```python
from build123d import *

# Parameters (mm, degrees)
SKETCH2_W            = 483.00005
SKETCH2_H            = 88.0999
BOSS_EXTRUDE2_DEPTH  = 3.0988
SKETCH3_W            = 163.4007
SKETCH3_H            = 30.8991
CUT_EXTRUDE1_DEPTH   = 3.0988
SKETCH5_R            = 2.5
CUT_EXTRUDE2_DEPTH   = 9.1948
LPATTERN1_COUNT      = 6
LPATTERN1_PITCH      = 20.32
LPATTERN1_COUNT_DIR2 = 4
LPATTERN1_PITCH_DIR2 = 10.16
SKETCH6_R            = 6.5024
CUT_EXTRUDE3_DEPTH   = 9.1948
LPATTERN2_COUNT      = 8
LPATTERN2_PITCH      = 20.32
SKETCH7_R            = 6.5024
CUT_EXTRUDE4_DEPTH   = 491.978862316
SKETCH8_R            = 5.92074
CUT_EXTRUDE5_DEPTH   = 491.978862316
SKETCH9_R            = 1.999996
CUT_EXTRUDE6_DEPTH   = 491.978862316
LPATTERN3_COUNT      = 6
LPATTERN3_PITCH      = 20.32
SKETCH10_R           = 2.5
CUT_EXTRUDE7_DEPTH   = 491.978862316
LPATTERN4_COUNT      = 2
LPATTERN4_PITCH      = 25.4
LPATTERN4_COUNT_DIR2 = 4
LPATTERN4_PITCH_DIR2 = 15.24
SKETCH11_R           = 1.999996
CUT_EXTRUDE8_DEPTH   = 491.978862316
LPATTERN5_COUNT      = 4
LPATTERN5_PITCH      = 10.16
SKETCH12_R           = 1.75
CUT_EXTRUDE9_DEPTH   = 491.978862316
LPATTERN6_COUNT      = 2
LPATTERN6_PITCH      = 12.7
LPATTERN6_COUNT_DIR2 = 2
LPATTERN6_PITCH_DIR2 = 25.4
SKETCH13_R           = 1.999996
CUT_EXTRUDE10_DEPTH  = 491.978862316
SKETCH15_R           = 5.92074
CUT_EXTRUDE11_DEPTH  = 491.978862316
LPATTERN7_COUNT      = 4
LPATTERN7_PITCH      = 38.1
SKETCH16_R           = 1.4732
CUT_EXTRUDE12_DEPTH  = 491.978862316
SKETCH17_R           = 1.4732
CUT_EXTRUDE13_DEPTH  = 491.978862316
SKETCH18_R           = 1.4732
CUT_EXTRUDE14_DEPTH  = 491.978862316


with BuildPart() as part:
    # Sketch2 → Boss-Extrude2 (new body)
    with BuildSketch(Plane.XY):
        with Locations((241.500025, 44.04995)):
            Rectangle(SKETCH2_W, SKETCH2_H)
    extrude(amount=-BOSS_EXTRUDE2_DEPTH)

    # Sketch3 → Cut-Extrude1 (cut)
    with BuildSketch(Plane.XY):
        with Locations((175.887888, 65.19037)):
            Rectangle(SKETCH3_W, SKETCH3_H)
    extrude(amount=-CUT_EXTRUDE1_DEPTH, mode=Mode.SUBTRACT)

    # Sketch5 → Cut-Extrude2 (cut)
    with BuildSketch(Plane.XY):
        with Locations((310.52008, 75.3999)):
            Circle(SKETCH5_R)
    cut_extrude2 = extrude(amount=-CUT_EXTRUDE2_DEPTH, mode=Mode.SUBTRACT)

    # LPattern1: Cut-Extrude2 6 × 4
    with Locations(*[(i * LPATTERN1_PITCH, -j * LPATTERN1_PITCH_DIR2, 0) for i in range(LPATTERN1_COUNT) for j in range(LPATTERN1_COUNT_DIR2) if (i, j) != (0, 0)]):
        add(cut_extrude2, mode=Mode.SUBTRACT)

    # Sketch6 → Cut-Extrude3 (cut)
    with BuildSketch(Plane.XY):
        with Locations((104.78008, 30.48)):
            Circle(SKETCH6_R)
    cut_extrude3 = extrude(amount=-CUT_EXTRUDE3_DEPTH, mode=Mode.SUBTRACT)

    # LPattern2: Cut-Extrude3 ×8
    with Locations(*[(i * LPATTERN2_PITCH, 0, 0) for i in range(1, LPATTERN2_COUNT)]):
        add(cut_extrude3, mode=Mode.SUBTRACT)

    # Sketch7 → Cut-Extrude4 (cut, through all)
    with BuildSketch(Plane.XY):
        with Locations((57.15, 48.26)):
            Circle(SKETCH7_R)
        with Locations((57.15, 33.02)):
            Circle(SKETCH7_R)
        with Locations((57.15, 17.78)):
            Circle(SKETCH7_R)
        with Locations((57.15, 63.5)):
            Circle(SKETCH7_R)
        with Locations((175.90008, 15.24)):
            Circle(SKETCH7_R)
        with Locations((280.66238, 30.48)):
            Circle(SKETCH7_R)
    extrude(amount=-CUT_EXTRUDE4_DEPTH, mode=Mode.SUBTRACT)

    # Sketch8 → Cut-Extrude5 (cut, through all)
    with BuildSketch(Plane.XY):
        with Locations((314.72505, 19.05)):
            Circle(SKETCH8_R)
    cut_extrude5 = extrude(amount=-CUT_EXTRUDE5_DEPTH, mode=Mode.SUBTRACT)

    # Sketch9 → Cut-Extrude6 (cut, through all)
    with BuildSketch(Plane.XY):
        with Locations((310.52008, 34.29)):
            Circle(SKETCH9_R)
    cut_extrude6 = extrude(amount=-CUT_EXTRUDE6_DEPTH, mode=Mode.SUBTRACT)

    # LPattern3: Cut-Extrude6 ×6
    with Locations(*[(i * LPATTERN3_PITCH, 0, 0) for i in range(1, LPATTERN3_COUNT)]):
        add(cut_extrude6, mode=Mode.SUBTRACT)

    # Sketch10 → Cut-Extrude7 (cut, through all)
    with BuildSketch(Plane.XY):
        with Locations((44.45, 63.5)):
            Circle(SKETCH10_R)
    cut_extrude7 = extrude(amount=-CUT_EXTRUDE7_DEPTH, mode=Mode.SUBTRACT)

    # LPattern4: Cut-Extrude7 2 × 4
    with Locations(*[(i * LPATTERN4_PITCH, -j * LPATTERN4_PITCH_DIR2, 0) for i in range(LPATTERN4_COUNT) for j in range(LPATTERN4_COUNT_DIR2) if (i, j) != (0, 0)]):
        add(cut_extrude7, mode=Mode.SUBTRACT)

    # Sketch11 → Cut-Extrude8 (cut, through all)
    with BuildSketch(Plane.XY):
        with Locations((432.44008, 75.3999)):
            Circle(SKETCH11_R)
    cut_extrude8 = extrude(amount=-CUT_EXTRUDE8_DEPTH, mode=Mode.SUBTRACT)

    # LPattern5: Cut-Extrude8 ×4
    with Locations(*[(0, -i * LPATTERN5_PITCH, 0) for i in range(1, LPATTERN5_COUNT)]):
        add(cut_extrude8, mode=Mode.SUBTRACT)

    # Sketch12 → Cut-Extrude9 (cut, through all)
    with BuildSketch(Plane(origin=(0, 0, -3.0988), x_dir=(-1, 0, 0), z_dir=(0, 0, -1))):
        with Locations((-260.887888, 78.44037)):
            Circle(SKETCH12_R)
        with Locations((-260.887888, 51.94037)):
            Circle(SKETCH12_R)
        with Locations((-85.887888, 78.44037)):
            Circle(SKETCH12_R)
        with Locations((-85.887888, 51.94037)):
            Circle(SKETCH12_R)
    extrude(amount=-CUT_EXTRUDE9_DEPTH, mode=Mode.SUBTRACT)

    # LPattern6: Cut-Extrude7 2 × 2
    with Locations(*[(j * LPATTERN6_PITCH_DIR2, i * LPATTERN6_PITCH, 0) for i in range(LPATTERN6_COUNT) for j in range(LPATTERN6_COUNT_DIR2) if (i, j) != (0, 0)]):
        add(cut_extrude7, mode=Mode.SUBTRACT)

    # Sketch13 → Cut-Extrude10 (cut, through all)
    with BuildSketch(Plane.XY):
        with Locations((57.15, 76.2)):
            Circle(SKETCH13_R)
    extrude(amount=-CUT_EXTRUDE10_DEPTH, mode=Mode.SUBTRACT)

    # Sketch15 → Cut-Extrude11 (cut, through all)
    with BuildSketch(Plane.XY):
        with Locations((276.23008, 65.19037)):
            Circle(SKETCH15_R)
    extrude(amount=-CUT_EXTRUDE11_DEPTH, mode=Mode.SUBTRACT)

    # LPattern7: Cut-Extrude5 ×4
    with Locations(*[(i * LPATTERN7_PITCH, 0, 0) for i in range(1, LPATTERN7_COUNT)]):
        add(cut_extrude5, mode=Mode.SUBTRACT)

    # Sketch16 → Cut-Extrude12 (cut, through all)
    with BuildSketch(Plane.XY):
        with Locations((28.575, 12.7)):
            Circle(SKETCH16_R)
        with Locations((28.575, 76.2)):
            Circle(SKETCH16_R)
    extrude(amount=-CUT_EXTRUDE12_DEPTH, mode=Mode.SUBTRACT)

    # Sketch17 → Cut-Extrude13 (cut, through all)
    with BuildSketch(Plane.XY):
        with Locations((291.846, 74.168)):
            Circle(SKETCH17_R)
        with Locations((290.576, 13.462)):
            Circle(SKETCH17_R)
    extrude(amount=-CUT_EXTRUDE13_DEPTH, mode=Mode.SUBTRACT)

    # Sketch18 → Cut-Extrude14 (cut, through all)
    with BuildSketch(Plane.XY):
        with Locations((124.714, 44.45)):
            Circle(SKETCH18_R)
        with Locations((220.98, 44.45)):
            Circle(SKETCH18_R)
    extrude(amount=-CUT_EXTRUDE14_DEPTH, mode=Mode.SUBTRACT)


solid = part.part
```
Geometry: final body of the model. Coordinates: model frame, mm. Round coordinates to 2 decimals unless told otherwise and drop trailing zeros. Loops run counter-clockwise (first coordinate to the right, second up) from the corner with the lowest first, then second, coordinate; pieces in that order, holes last. Notation, with made-up numbers: (25.25, 35) -> (74.25, 35) arc R14 ccw to (74.25, 59) -> close; hole circle Ø3 at (50, 8). An arc over 180 degrees is marked (long way). Use one line per item in the form item = value. Start each with the question number.
1) Section A-A on x = 103.5. Output: boundary loops of the cut face in (y, z).
2) Section B-B on z = -0.6. Give the number of separate pieces and of enclosed holes in the cut face, then the cut area to 3 significant figures.
3) Section C-C on x = 187.5. Output: boundary loops of the cut face in (y, z), then the cut area to 3 significant figures.
4) First-contact query: P1, Ø4.5, axis at x = 371.48, y = 55.08, coming from the +Z side; P2, Ø6.5, axis at x = 310.52, y = 65.24, coming from the -Z side. Flat tips, straight axial feed; report the tip coordinate or a pass-through.
5) Draft query along X for faces 1 (the flat face through (238, 45, 0)), 2 (the cylindrical face through (281.877, 66.969, -1.528)). Return one class per face: released by +X, released by -X, zero draft, split by the parting line, or undercut.
6) Line query: L1, parallel to Y at x = 44.45, z = -1.5; L2, parallel to X at y = 79, z = -0.1; L3, parallel to Y at x = 185.5, z = -2.35. Output: solid intervals per line, ascending.
Response:
q1.outline = (0, -3.1) -> (24.1, -3.1) -> (24.1, 0) -> (0, 0) -> close; (36.86, -3.1) -> (49.74, -3.1) -> (49.74, 0) -> (36.86, 0) -> close; (80.64, -3.1) -> (88.1, -3.1) -> (88.1, 0) -> (80.64, 0) -> close
q2.separate_pieces = 1
q2.enclosed_holes = 75
q2.area = 34,200 mm^2
q3.outline = (0, -3.1) -> (24.14, -3.1) -> (24.14, 0) -> (0, 0) -> close; (36.82, -3.1) -> (49.74, -3.1) -> (49.74, 0) -> (36.82, 0) -> close; (80.64, -3.1) -> (88.1, -3.1) -> (88.1, 0) -> (80.64, 0) -> close
q3.area = 138 mm^2
q4.P1 = through
q4.P2 = -3.1
q5.face_1 = zero draft
q5.face_2 = undercut
q6.L1 = 0 to 15.28, 20.28 to 30.52, 35.52 to 45.76, 50.76 to 61, 66 to 73.7, 78.7 to 88.1
q6.L2 = 0 to 84.23, 87.55 to 94.19, 257.59 to 259.23, 262.55 to 483
q6.L3 = 0 to 24, 36.96 to 49.74, 80.64 to 88.1
